Input: part model. Units: mm. Frame: model coordinates. A direction names the side the tool comes from. Round coordinates to 2 decimals unless told otherwise and drop trailing zeros. Loops run counter-clockwise (first coordinate to the right, second up) from the corner with the lowest first, then second, coordinate; pieces in that order, holes last. Notation, with made-up numbers: (-30.75, 79.5) - (14.25, 79.5) arc R21 cw to (14.25, 113.5) - close; hole circle Ø11 at (-31, 69.25). An arc over 180 degrees is marked (long way). One line per question, with ' | ' between items. Start each with the question number.
Item 1: Section A-A, the plane z = 2.5. Return loops of the section in (x, y).
Item 2: Material intervals for line 1 along Z through (x, y) = (0.5, -1); line 2 along Z through (x, y) = (-0.75, -2); line 3 along Y through (x, z) = (0.75, -15), sorted ascending.
Item 3: Set-up query: faces 1 (the face through (0, 0, -24)), 2 (the face through (-2, -1, 6)). Return all of +Z, -Z, +X, -X, +Y, -Y with unobstructed straight access to the full face (end or side cutting, diameter ignored); none if empty.
Item 4: First-contact query: pin 1 (2 mm diameter, centred on x = 0, z = -2.5, fed in from -Y); pin 2 (3 mm diameter, centred on x = 3, z = -4, fed in from +Y); pin 3 (4 mm diameter, centred on y = 2, z = 2.5, fed in from +X). Flat tips, straight axial feed; report the tip coordinate or a pass-through.
Autodesk Inventor part; units mm, degrees
ref_plane "YZ Plane" through (0, 0, 0) normal (1, 0, 0) x (0, 1, 0)
ref_plane "XZ Plane" through (0, 0, 0) normal (0, 1, 0) x (-1, 0, 0)
ref_plane "XY Plane" through (0, 0, 0) normal (0, 0, 1) x (1, 0, 0)
sketch "スケッチ1" plane through (0, 0, 0) normal (0, 0, 1) x (1, 0, 0)
  circle A0 centre (0, 0) radius 2
  dimension "d0" = 4
extrude "押し出し1" add sketch "スケッチ1" along normal blind 6
sketch "スケッチ2" plane through (0, 0, 6) normal (0, 0, 1) x (1, 0, 0)
  circle A0 centre (0, 0) radius 2
  circle A1 centre (0, 0) radius 4
  dimension "d3" = 8
extrude "押し出し2" add sketch "スケッチ2" along normal blind 3 contours A0 | A1
fillet "フィレット1" radius 3 1 edges at (-4, 0, 9)
thread "ねじ1"
sketch "スケッチ3" plane through (0, 0, 0) normal (0, 0, -1) x (-1, 0, 0)
  circle A0 centre (0, 0) radius 2
extrude "押し出し3" add sketch "スケッチ3" along normal blind 24
properties part number "SB　M4 30mm なべネジ" material "Stainless Steel, 440C"
Return value:
1) outline: circle Ø4 at (0, 0)
2) line 1: -24 to 9 | line 2: 6 to 8.78 | line 3: -1.85 to 1.85
3) face 1: -Z, +X, -X, +Y, -Y | face 2: -Z
4) pin 1: y = -2 | pin 2: y = 1.32 | pin 3: x = 2
